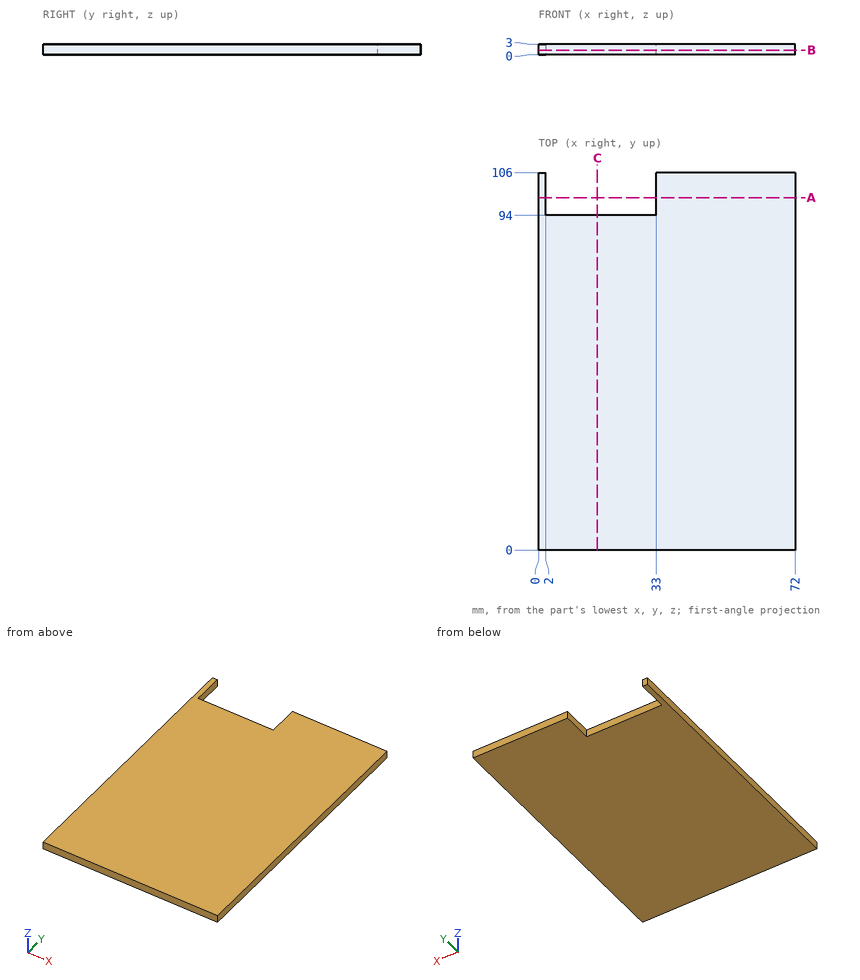
Answer from the drawing. Dimensions are ordinates in mm from the lowest x, y and z of the part. Give positions to 0.01 mm unless a question says otherwise; leave off trailing zeros. Order: outer loops, then holes, each group sorted by start corner. A loop starts at its lowest first (then second) coordinate and runs counter-clockwise, first axis right, second up. Notation, with made-up numbers: (78, 59.5) -> (123, 59.5) arc R16 cw to (123, 70.5) -> close; hole circle Ø6 at (12.25, 73). An arc over 180 degrees is marked (long way). One line per item, written item: value. Start each with the question number.
(1) The part is cut by section C-C (x = 16.5). Determine the outline of the cut face in (y, z), and give its area (3 significant figures).
(2) The part is cut by section B-B (z = 1.3). Determine the outline of the cut face in (x, y).
(3) Straight lines are drawn through the part: L1, parallel to X at y = 98, z = 0.6; L2, parallel to Y at x = 16, z = 1.55. For each, find the intervals that lie inside material, in ascending order.
(4) The part is cut by section A-A (y = 99). Determine the outline of the cut face in (x, z), and give its area (3 significant figures).
(5) A flat-ended cylindrical pin translates along its axis: P1, Ø1.5, axis at x = 24.5, z = 2, coming from the +Y side. Find the tip coordinate at first contact, or state that the pin passes through.
Taken from the geometry:
1. outline: (0, 0) -> (94, 0) -> (94, 3) -> (0, 3) -> close
1. area: 282 mm^2
2. outline: (0, 0) -> (72, 0) -> (72, 106) -> (33, 106) -> (33, 94) -> (2, 94) -> (2, 106) -> (0, 106) -> close
3. L1: 0 to 2, 33 to 72
3. L2: 0 to 94
4. outline: (0, 0) -> (2, 0) -> (2, 3) -> (0, 3) -> close; (33, 0) -> (72, 0) -> (72, 3) -> (33, 3) -> close
4. area: 123 mm^2
5. P1: y = 94
